Can you work these out from the model? Positions are in its coordinate system, mm. A direction names the side the tool comes from. Coordinates: 2 decimals unless noted, no trailing zeros. Loops run counter-clockwise (first coordinate to the right, second up) from the corner with the lowest first, then second, coordinate; pieces in that order, holes last.
```python
from build123d import *

# Parameters (mm, degrees)
SKETCH075_R     = 49.5
SKETCH075_R_2   = 1.6
PAD039_DEPTH    = 7.5
SKETCH076_R     = 19
SKETCH076_R_2   = 6
POCKET036_DEPTH = 2.5
CHAMFER012_SIZE = 1
CHAMFER013_SIZE = 0.4


with BuildPart() as part:
    # Sketch075 → Pad039 (new body)
    with BuildSketch(Plane.XY):
        Circle(SKETCH075_R)
        with Locations((0, 33)):
            Circle(SKETCH075_R_2, mode=Mode.SUBTRACT)
        with Locations((28.578838, -16.5)):
            Circle(SKETCH075_R_2, mode=Mode.SUBTRACT)
        with Locations((-28.578838, -16.5)):
            Circle(SKETCH075_R_2, mode=Mode.SUBTRACT)
    extrude(amount=-PAD039_DEPTH)

    # Sketch076 (on Face6 of Pad039) → Pocket036 (cut)
    with BuildSketch(Plane(origin=(0, 0, -7.5), x_dir=(1, 0, 0), z_dir=(0, 0, -1))):
        Circle(SKETCH076_R)
        with Locations((28.578838, 16.5)):
            Circle(SKETCH076_R_2)
        with Locations((0, -33)):
            Circle(SKETCH076_R_2)
        with Locations((-28.578838, 16.5)):
            Circle(SKETCH076_R_2)
    extrude(amount=-POCKET036_DEPTH, mode=Mode.SUBTRACT)

    # Chamfer012
    chamfer012_edges = [part.edges().sort_by_distance(p)[0] for p in [
        (-19, 0, -7.5),
        (22.578838, -16.5, -7.5),
        (-34.578838, -16.5, -7.5),
        (-6, 33, -7.5),
        (-49.5, 0, -7.5),
    ]]
    chamfer(chamfer012_edges, length=CHAMFER012_SIZE)

    # Chamfer013
    chamfer013_edges = [part.edges().sort_by_distance(p)[0] for p in [
        (26.978838, -16.5, -5),
        (-1.6, 33, -5),
        (-1.6, 33, 0),
        (26.978838, -16.5, 0),
        (-30.178838, -16.5, -5),
        (-30.178838, -16.5, 0),
        (-49.5, 0, 0),
    ]]
    chamfer(chamfer013_edges, length=CHAMFER013_SIZE)


with BuildPart() as part_1:
    # Body033 placement: moved
    add(part.part.moved(Location((0, 0, 92))))


solid = part_1.part
```
Item 1: We'd pull the mould along Y, two halves only. Please class faces 1 (the face through (-0.35, 31.44, 89.53)), 2 (the face through (21, 1, 84.5)), 3 (the face through (-6.44, 49.08, 88.59)): +Y half, -Y half, draft (parallel to the pull), parting line (faces both ways), or undercut.
Results are:
face 1: undercut
face 2: draft
face 3: parting line
Item 2: I need wall thicknesses on line 1 along Y through (x, z) = (0, 90.2); line 2 along X through (y, z) = (-16.5, 86.7); line 3 along Z through (x, y) = (4, 16). Which ranges of each line are inside material? Lowest first, please.
Results are:
line 1: y = -49.5 to 31.4, 34.6 to 49.5
line 2: x = -46.67 to -34.58, -22.58 to -9.42, 9.42 to 22.58, 34.58 to 46.67
line 3: z = 87 to 92
Item 3: On a 3-axis mill with a long thin cutter (end or side, diameter ignored), from which of +Z, -Z, +X, -X, +Y, -Y can I reach the whole of each face in a straight line? I mean faces 4 (the face through (27.4, -15.42, 89.53)), 5 (the face through (-1.301, 38.857, 86.239)). Say none if no direction works.
Results are:
face 4: +Z, -Z
face 5: -Z
Item 4: Suppose I cut it at B-B, the plane y = 0. Please give me the cut outline in (x, z), plus the area to 3 significant figures.
Results are:
outline: (-49.5, 85.5) - (-48.5, 84.5) - (-20, 84.5) - (-19, 85.5) - (-19, 87) - (19, 87) - (19, 85.5) - (20, 84.5) - (48.5, 84.5) - (49.5, 85.5) - (49.5, 91.6) - (49.1, 92) - (-49.1, 92) - (-49.5, 91.6) - close
area: 645 mm2
Item 5: I'm going to push flat-ended pins straight in: P1, Ø9.5, axis at x = -1, y = 33, coming from the -Z side; P2, Ø1.5, axis at y = -29, z = 85.5, coming from the -X side; P3, Ø2, axis at x = 6.5, z = 85.5, coming from the -Y side. Where does each tip first touch, or does it pass through?
Results are:
P1: stops at z = 87
P2: stops at x = -40.65
P3: stops at y = -49.19
Item 6: Suppose I cut it at C-C, the plane z = 89.25. Please give me the cut outline in (x, y).
Results are:
outline: circle Ø99 at (0, 0); hole circle Ø3.2 at (-28.58, -16.5); hole circle Ø3.2 at (0, 33); hole circle Ø3.2 at (28.58, -16.5)
Item 7: Suppose I cut it at A-A, the plane x = 0. Please give me the cut outline in (y, z), plus the area to 3 significant figures.
Results are:
outline: (-49.5, 85.5) - (-48.5, 84.5) - (-20, 84.5) - (-19, 85.5) - (-19, 87) - (19, 87) - (19, 85.5) - (20, 84.5) - (26, 84.5) - (27, 85.5) - (27, 87) - (31, 87) - (31.4, 87.4) - (31.4, 91.6) - (31, 92) - (-49.1, 92) - (-49.5, 91.6) - close; (34.6, 87.4) - (35, 87) - (39, 87) - (39, 85.5) - (40, 84.5) - (48.5, 84.5) - (49.5, 85.5) - (49.5, 91.6) - (49.1, 92) - (35, 92) - (34.6, 91.6) - close
area: 598 mm2
